Read the model definition and answer for the solid it produces. Units are mm, in the model's axes. Give positions to 0.01 mm unless a question says otherwise; leave off trailing zeros. Loops run counter-clockwise (first coordinate to the right, second up) from the corner with the lowest first, then second, coordinate; pieces in that order, holes last. Notation, with made-up numbers: (20, 32) - (76, 32) arc R11 ccw to (76, 43) - close; hole circle Ø9 at (-32, -34). An arc over 180 degrees is marked (long way). Write item = value, one per line. Start each with the question number.
from build123d import *

# Parameters (mm, degrees)
F0_W     = 19.05
F0_H     = 19.05
F1_DEPTH = 9.525
F2_R     = 3.302
F3_DEPTH = 3.683


with BuildPart() as f1:
    # F0 (on Top) → F1 (new body, symmetric)
    with BuildSketch(Plane.XY):
        Rectangle(F0_W, F0_H)
    extrude(amount=F1_DEPTH, both=True)

    # F2 (on face) → F3 (cut)
    with BuildSketch(Plane(origin=(0, 0, -9.525), x_dir=(1, 0, 0), z_dir=(0, 0, -1))):
        Circle(F2_R)
    extrude(amount=-F3_DEPTH, mode=Mode.SUBTRACT)


solid = f1.part
1. A cutting plane is placed at A-A on x = 0. Give the vertices of the cut face in (y, z) (3 decimals), and give its area (3 significant figures).
2. Consider line 1 along X through (y, z) = (0, -8.7) (3 decimals); line 2 along Z through (x, y) = (2, -1.25) (3 decimals). Determine where each line is inside the solid, lowest interval first. Write a range as [from, to].
3. A cutting plane is placed at B-B on z = -7.25. Give the vertices of the cut face in (x, y) (3 decimals).
4. Given P1, Ø3.5, axis at x = -0.5, y = -0.5, coming from the -Z side, flat-ended and moving along its own axis, determine where the tip first touches the part or whether it passes through.
5. For a pull along X with two mould halves and no side action, classify faces 1 (the flat face through (0, 0, 9.525)), 2 (the flat face through (0, 0, -5.842)), 3 (the cylindrical face through (3.05, 1.26, -7.71)), 4 (the flat face through (-9.525, 0, 0)) as released by +X, released by -X, zero draft, split by the parting line, or undercut.
Reply:
q1.outline = (-9.525, -9.525) - (-3.302, -9.525) - (-3.302, -5.842) - (3.302, -5.842) - (3.302, -9.525) - (9.525, -9.525) - (9.525, 9.525) - (-9.525, 9.525) - close
q1.area = 339 mm^2
q2.line_1 = [-9.525, -3.302], [3.302, 9.525]
q2.line_2 = [-5.842, 9.525]
q3.outline = (-9.525, -9.525) - (9.525, -9.525) - (9.525, 9.525) - (-9.525, 9.525) - close; hole circle Ø6.604 at (0, 0)
q4.P1 = -5.84
q5.face_1 = zero draft
q5.face_2 = undercut
q5.face_3 = undercut
q5.face_4 = released by -X
